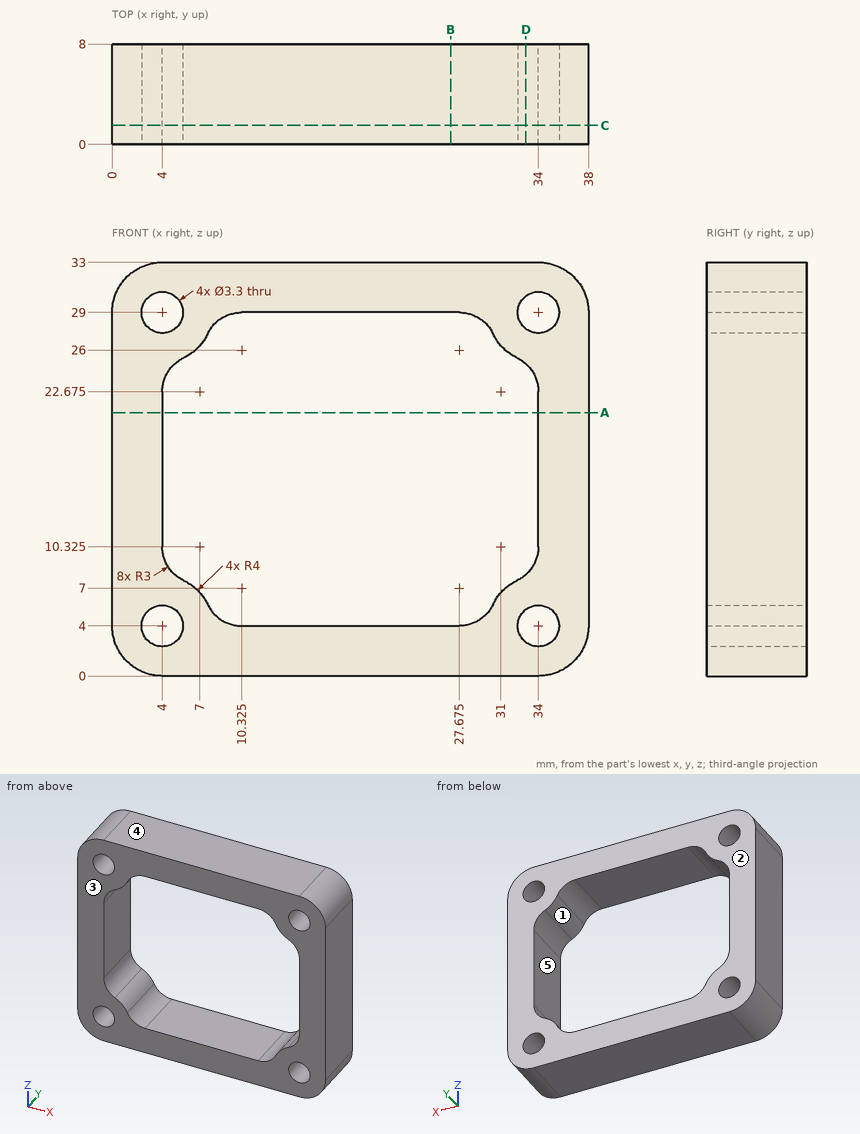
Can you work these out from the drawing? Everything is in mm from the part's minimum corner. A direction names the side the tool comes from. Coordinates: 2 decimals unless noted, no trailing zeros. Write each loop counter-clockwise with the first axis right and the second up, starting at its lowest first coordinate (ties: lowest second). Pieces come first, ordered by that corner, then holes. Notation, with made-up numbers: (78.25, -29.75) - (130.25, -29.75) arc R21 cw to (130.25, -1.75) - close; hole circle Ø2 at (52, 58). An arc over 180 degrees is marked (long way). One line per item, written item: value.
1) On a 3-axis mill with a long thin cutter (end or side, diameter ignored), from which of +Z, -Z, +X, -X, +Y, -Y can I reach the whole of each face in a straight line? I mean the marked faces 1 and 2. Say none if no direction works.
Model answer:
face 1: +Y, -Y
face 2: +Z, -Z, +X, -X, +Y
2) We'd pull the mould along Z, two halves only. Please class the marked faces 3, 4 and 5: pulls with the +Z half, pulls with the -Z half, needs draft (parallel to the pull), parting line crosses it, or undercut.
Model answer:
face 3: needs draft
face 4: pulls with the +Z half
face 5: undercut
3) Suppose I cut it at B-B on x = 27. Write out the boundary of the cut face in (y, z).
Model answer:
outline: (0, 0) - (8, 0) - (8, 4) - (0, 4) - close; (0, 29) - (8, 29) - (8, 33) - (0, 33) - close
4) Suppose I cut it at A-A on z = 21. Write out the boundary of the cut face in (x, y), and give its area (3 significant figures).
Model answer:
outline: (0, 0) - (4, 0) - (4, 8) - (0, 8) - close; (34, 0) - (38, 0) - (38, 8) - (34, 8) - close
area: 64.0 mm²
5) I need wall thicknesses on line 1 along Z through (x, y) = (16.5, 1.75); line 2 along X through (y, z) = (2.5, 15.5); line 3 along Z through (x, y) = (3.5, 2.5). Which ranges of each line are inside material? Lowest first, please.
Model answer:
line 1: z = 0 to 4, 29 to 33
line 2: x = 0 to 4, 34 to 38
line 3: z = 0.03 to 2.43, 5.57 to 27.43, 30.57 to 32.97
6) Suppose I cut it at D-D on x = 33. Write out the boundary of the cut face in (y, z).
Model answer:
outline: (0, 0) - (8, 0) - (8, 2.69) - (0, 2.69) - close; (0, 5.31) - (8, 5.31) - (8, 8.09) - (0, 8.09) - close; (0, 24.91) - (8, 24.91) - (8, 27.69) - (0, 27.69) - close; (0, 30.31) - (8, 30.31) - (8, 33) - (0, 33) - close
7) Suppose I cut it at C-C on y = 1.5. State how many separate pieces and enclosed holes the cut face has.
Model answer:
separate pieces: 1
enclosed holes: 5
